Input: part model. Units: mm. Frame: model coordinates. Face numbers are marked on the shaded views. A direction names the side the tool comes from. Coordinates: 2 decimals unless noted, no trailing zeros. Write each loop counter-clockwise with the first axis right and the second up, starting at its lowest first coordinate (ties: lowest second). Pieces come first, ordered by that corner, then holes. Notation, with made-up numbers: (32, 38) - (64, 38) arc R26 ccw to (64, 77) - close; hole circle Ø2 at (-34.5, -16). An arc over 180 degrees is marked (long way). Use a Markdown table: item, result. Add a question column.
Q1. Set-up query: the marked faces 1 and 2. Return all of +Z, -Z, +X, -X, +Y, -Y with unobstructed straight access to the full face (end or side cutting, diameter ignored); none if empty.
Q2. Section query C-C (y = 3.5). Give the number of separate pieces and of enclosed holes in the cut face, then the cut area to 3 significant figures.
Q3. Section query A-A (x = 0). Return the cut outline in (y, z), then the cut area to 4 significant figures.
Q4. Material intervals for probe 1 along Z at (x, y) = (-18, 2); probe 2 along Z at (x, y) = (-78, 2.5); probe 3 along X at (y, z) = (-4, 4.5), sorted ascending. Write a range as from..to.
Q5. Pin query (flat end, axial travel): P1, Ø4, axis at x = -35.5, y = 1, coming from the -Z side; P2, Ø3, axis at x = 0, y = 0, coming from the -Z side; P3, Ø1.5, axis at x = 7, y = 1, coming from the -Z side; P4, Ø2, axis at y = -0.5, z = 7.5, coming from the +X side. Return the tip coordinate at first contact, or that it passes through.
Q6. Section query D-D (x = -18). Return the cut outline in (y, z), then the cut area to 3 significant figures.
Q7. Section query B-B (z = 10). Return the cut outline in (x, y), then the cut area to 3 significant figures.
from build123d import *

# Parameters (mm, degrees)
SKETCH1_W                  = 10
SKETCH1_H                  = 10
BOSS_EXTRUDE1_DEPTH        = 11
SKETCH2_W                  = 2
SKETCH2_H                  = 10
BOSS_EXTRUDE2_DEPTH        = 3
BOSS_EXTRUDE2_DEPTH_BACK   = 13
SKETCH3_W                  = 40
SKETCH3_H                  = 10
BOSS_EXTRUDE3_DEPTH        = 10
SKETCH5_W                  = 10
SKETCH5_H                  = 10
BOSS_EXTRUDE4_DEPTH        = 70
F_2_5MM_DOWEL_SLOT1_D      = 2.5
F_3_2_3_2_DIAMETER_SLOT2_D = 3.2


with BuildPart() as part:
    # Sketch1 → Boss-Extrude1 (new body)
    with BuildSketch(Plane.XY):
        Rectangle(SKETCH1_W, SKETCH1_H)
    extrude(amount=BOSS_EXTRUDE1_DEPTH)

    # Sketch2 → Boss-Extrude2 (add, two sides)
    with BuildSketch(Plane(origin=(5, 0, 0), x_dir=(0, 0, -1), z_dir=(1, 0, 0))) as boss_extrude2_sk:
        with Locations((-2.5, 0)):
            Rectangle(SKETCH2_W, SKETCH2_H)
    extrude(amount=BOSS_EXTRUDE2_DEPTH)
    extrude(boss_extrude2_sk.sketch, amount=-BOSS_EXTRUDE2_DEPTH_BACK)

    # Sketch3 → Boss-Extrude3 (add)
    with BuildSketch(Plane.XY.offset(11)):
        Rectangle(SKETCH3_W, SKETCH3_H)
    extrude(amount=BOSS_EXTRUDE3_DEPTH)

    # Sketch5 → Boss-Extrude4 (add)
    with BuildSketch(Plane.ZY.offset(20)):
        with Locations((16, 0)):
            Rectangle(SKETCH5_W, SKETCH5_H)
    extrude(amount=BOSS_EXTRUDE4_DEPTH)

    # Ø2.5mm Dowel Slot1 (through all)
    with Locations(Plane.XY.offset(21)):
        with Locations((0, 0)):
            Hole(F_2_5MM_DOWEL_SLOT1_D / 2)

    # Ø3.2 (3.2) Diameter Slot2 (through all)
    with Locations(Plane(origin=(0, -5, 0), x_dir=(-1, 0, 0), z_dir=(0, -1, 0))):
        with Locations((85, -16.229165357), (80, -16.229165357), (48, -16.229165357), (43, -16.229165357), (75, -16.229165357), (70, -16.229165357), (65, -16.229165357), (60, -16.229165357), (38, -16.229165357), (33, -16.229165357), (28, -16.229165357), (23, -16.229165357), (55, -16.229165357), (18, -16.229165357)):
            Hole(F_3_2_3_2_DIAMETER_SLOT2_D / 2)


solid = part.part
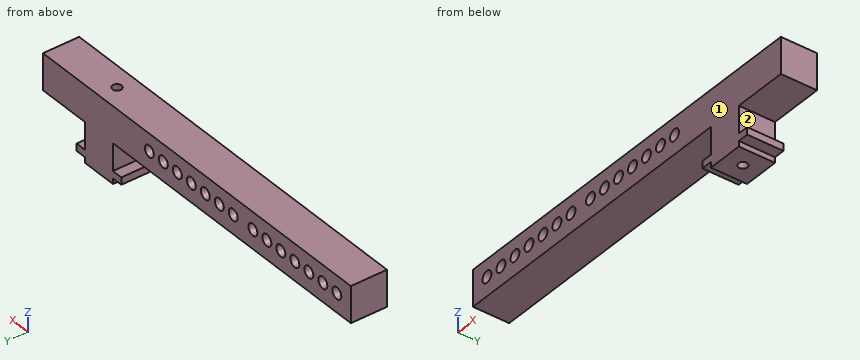
Values follow:
| question | item | result |
|---|---|---|
| 1 | face 1 | +Z, -Z, +X, -X, -Y |
| 1 | face 2 | +X, +Y, -Y |
| 2 | separate pieces | 1 |
| 2 | enclosed holes | 14 |
| 2 | area | 1,110 mm2 |
| 3 | outline | (-5, 0) - (-1.25, 0) - (-1.25, 21) - (-5, 21) - close; (1.25, 0) - (5, 0) - (5, 21) - (1.25, 21) - close |
| 3 | area | 157.5 mm2 |
| 4 | probe 1 | 11..14.63, 17.83..21 |
| 4 | probe 2 | 11..21 |
| 4 | probe 3 | -5..5 |
| 5 | P1 | z = 11 |
| 5 | P2 | z = 0 |
| 5 | P3 | z = 1.5 |
| 5 | P4 | x = 5 |
| 6 | outline | (-5, 11) - (5, 11) - (5, 14.63) - (-5, 14.63) - close; (-5, 17.83) - (5, 17.83) - (5, 21) - (-5, 21) - close |
| 6 | area | 68.0 mm2 |
| 7 | outline | (-5, -5) - (5, -5) - (5, 5) - (-5, 5) - close; hole circle Ø2.5 at (0, 0) |
| 7 | area | 95.1 mm2 |
